Part model, mm, in its own coordinate system. A direction names the side the tool comes from. Round coordinates to 2 decimals unless told otherwise and drop trailing zeros. Order: outer loops, then holes, each group sorted by start corner. A loop starts at its lowest first (then second) coordinate and runs counter-clockwise, first axis right, second up. Notation, with made-up numbers: M 30.5,-8 L 76.5,-8 A11 ccw 76.5,13 Z; hole C 69,-28.5 d1. An arc over 180 degrees is marked long. Write each question's results on one line, items separated by ' | '. Start each with the question number.
1. Band-saw the part on B-B, the plane z = 20.5. List the corners of the cut face in (x, y), then the cut area to 3 significant figures.
2. Which spindle directions (+Z, -Z, +X, -X, +Y, -Y) get a long thin tool onto all of the face, cutting with end or side? Do faces 1 (the face through (-260.57, -2, 19)), 2 (the face through (9, 3, 12.7)), 3 (the face through (9, 172.316, 19)). Say none if no direction does.
3. Band-saw the part on C-C, the plane x = 32. List the corners of the cut face in (y, z), then the cut area to 3 significant figures.
4. Two-plate mould, pull along Y, no slides. Class faces 4 (the face through (9, -176.934, 6)), 5 (the face through (9, 178.666, 6)), 6 (the face through (9, -164.234, 19)), 7 (the face through (9, 165.966, 19)): +Y half, -Y half, draft (parallel to the pull), parting line (faces both ways), or undercut.
5. Band-saw the part on A-A, the plane y = 53.5. List the corners of the cut face in (x, z).
6. Drop flat-ended pins along their axis: pin 1 Ø6.5 at (x, z) = (79, 20.5) entering from -Y; pin 2 Ø14 at (x, z) = (-121.5, 21) entering from +Y; pin 3 Ø10 at (y, z) = (-61, 18) entering from +X. Give the stop position or say it passes through.
7. Probe L1, parallel to Y at x = 34.5, z = 23; L2, parallel to X at y = 30.5, z = 15.5; L3, parallel to Z at x = -76.5, y = 87. List the from-to ranges inside material, lowest first. Write a range as [from, to].
```python
from build123d import *

# Parameters (mm, degrees)
F0_W     = 558.8
F0_H     = 355.6
F1_DEPTH = 25.4
F2_W     = 533.4
F2_H     = 330.2
F3_DEPTH = 12.7
F4_W     = 558.8
F4_H     = 355.6
F4_W_2   = 546.1
F4_H_2   = 342.9
F5_DEPTH = 12.7


with BuildPart() as f1:
    # F0 (on Top) → F1 (new body)
    with BuildSketch(Plane.XY):
        with Locations((12.479961, 0.865745)):
            Rectangle(F0_W, F0_H)
    extrude(amount=F1_DEPTH)

    # F2 (on face) → F3 (cut)
    with BuildSketch(Plane.XY.offset(25.4)):
        with Locations((12.479961, 0.865745)):
            Rectangle(F2_W, F2_H)
    extrude(amount=-F3_DEPTH, mode=Mode.SUBTRACT)

    # F4 (on face) → F5 (cut)
    with BuildSketch(Plane.XY.offset(25.4)):
        with Locations((12.479961, 0.865745)):
            Rectangle(F4_W, F4_H)
        with Locations((12.479961, 0.865745)):
            Rectangle(F4_W_2, F4_H_2, mode=Mode.SUBTRACT)
    extrude(amount=-F5_DEPTH, mode=Mode.SUBTRACT)


solid = f1.part
```
Solution:
1) outline: M -260.57,-170.58 L 285.53,-170.58 L 285.53,172.32 L -260.57,172.32 Z; hole M -254.22,-164.23 L 279.18,-164.23 L 279.18,165.97 L -254.22,165.97 Z | area: 11,100 mm^2
2) face 1: +Z, -X, +Y, -Y | face 2: +Z | face 3: +Z, +X, -X, +Y
3) outline: M -176.93,0 L 178.67,0 L 178.67,12.7 L 172.32,12.7 L 172.32,25.4 L 165.97,25.4 L 165.97,12.7 L -164.23,12.7 L -164.23,25.4 L -170.58,25.4 L -170.58,12.7 L -176.93,12.7 Z | area: 4,680 mm^2
4) face 4: -Y half | face 5: +Y half | face 6: undercut | face 7: undercut
5) outline: M -266.92,0 L 291.88,0 L 291.88,12.7 L 285.53,12.7 L 285.53,25.4 L 279.18,25.4 L 279.18,12.7 L -254.22,12.7 L -254.22,25.4 L -260.57,25.4 L -260.57,12.7 L -266.92,12.7 Z
6) pin 1: y = -170.58 | pin 2: y = 172.32 | pin 3: x = 285.53
7) L1: [-170.58, -164.23], [165.97, 172.32] | L2: [-260.57, -254.22], [279.18, 285.53] | L3: [0, 12.7]
